from build123d import *

# Parameters (mm, degrees)
F0_W     = 38.1
F0_H     = 38.1
F1_DEPTH = 6.35
F2_R     = 2.54
F3_DEPTH = 6.351
F4_R     = 9.525
F5_DEPTH = 6.351


with BuildPart() as f1:
    # F0 (on Front) → F1 (new body)
    with BuildSketch(Plane.XZ):
        Rectangle(F0_W, F0_H)
    extrude(amount=F1_DEPTH)

    # F2 (on face) → F3 (cut, through all)
    with BuildSketch(Plane.XZ.offset(6.35)):
        with Locations((-13.97, 13.97)):
            Circle(F2_R)
        with Locations((13.97, 13.97)):
            Circle(F2_R)
        with Locations((13.97, -13.97)):
            Circle(F2_R)
        with Locations((-13.97, -13.97)):
            Circle(F2_R)
    extrude(amount=-F3_DEPTH, mode=Mode.SUBTRACT)

    # F4 (on face) → F5 (cut, through all)
    with BuildSketch(Plane.XZ.offset(6.35)):
        Circle(F4_R)
    extrude(amount=-F5_DEPTH, mode=Mode.SUBTRACT)


solid = f1.part
Verification items for the finished model (mm, model axes). Round coordinates to 2 decimals unless told otherwise and drop trailing zeros. Loops run counter-clockwise (first coordinate to the right, second up) from the corner with the lowest first, then second, coordinate; pieces in that order, holes last. Notation, with made-up numbers: (-15, 23.25) - (21, 23.25) arc R15 ccw to (21, 46.25) - close; hole circle Ø2 at (-23, 85.25). An arc over 180 degrees is marked (long way). Write item = value, one per line.
Q1. Sectioned sample at B-B on x = 0. Record the boundary of the cut face in (y, z) (3 decimals).
Here are the results:
outline = (-6.35, -19.05) - (0, -19.05) - (0, -9.525) - (-6.35, -9.525) - close; (-6.35, 9.525) - (0, 9.525) - (0, 19.05) - (-6.35, 19.05) - close
Q2. Sectioned sample at D-D on z = 0. Record the boundary of the cut face in (x, y) (3 decimals).
Here are the results:
outline = (-19.05, -6.35) - (-9.525, -6.35) - (-9.525, 0) - (-19.05, 0) - close; (9.525, -6.35) - (19.05, -6.35) - (19.05, 0) - (9.525, 0) - close
Q3. Material ranges on L1, parallel to Z at x = -14, y = -1; L2, parallel to Z at x = 0, y = -3 (3 decimals); L3, parallel to X at y = -5.25, z = -12, recorded low to high.
Here are the results:
L1 = -19.05 to -16.51, -11.43 to 11.43, 16.51 to 19.05
L2 = -19.05 to -9.525, 9.525 to 19.05
L3 = -19.05 to -15.57, -12.37 to 12.37, 15.57 to 19.05
Q4. Depth check by flat-ended pin: pin 1 (3 mm diameter, centred on x = 13.97, z = 13.97, fed in from -Y). Enter the tip coordinate at first touch or a pass-through.
Here are the results:
pin_1 = through
Q5. Sectioned sample at A-A on z = 13.97. Record the boundary of the cut face in (x, y), plus the area to 3 significant figures.
Here are the results:
outline = (-19.05, -6.35) - (-16.51, -6.35) - (-16.51, 0) - (-19.05, 0) - close; (-11.43, -6.35) - (11.43, -6.35) - (11.43, 0) - (-11.43, 0) - close; (16.51, -6.35) - (19.05, -6.35) - (19.05, 0) - (16.51, 0) - close
area = 177 mm^2
Q6. Sectioned sample at C-C on y = -4. Record the boundary of the cut face in (x, z) (3 decimals), plus the area to 3 significant figures.
Here are the results:
outline = (-19.05, -19.05) - (19.05, -19.05) - (19.05, 19.05) - (-19.05, 19.05) - close; hole circle Ø5.08 at (-13.97, -13.97); hole circle Ø5.08 at (-13.97, 13.97); hole circle Ø19.05 at (0, 0); hole circle Ø5.08 at (13.97, -13.97); hole circle Ø5.08 at (13.97, 13.97)
area = 1,090 mm^2
Q7. Mould release check, pull along Z, two halves, no side actions. Record for faces 1 (the cylindrical face through (16.393, -3.219, 14.733)), 2 (the flat face through (0, -3, -19.05)), 3 (the cylindrical face through (15.142, -3.219, -16.223)), 4 (the flat face through (-5, -6.35, 9)): +Z half, -Z half, draft (parallel to the pull), parting line (faces both ways), or undercut.
Here are the results:
face_1 = undercut
face_2 = -Z half
face_3 = undercut
face_4 = draft
